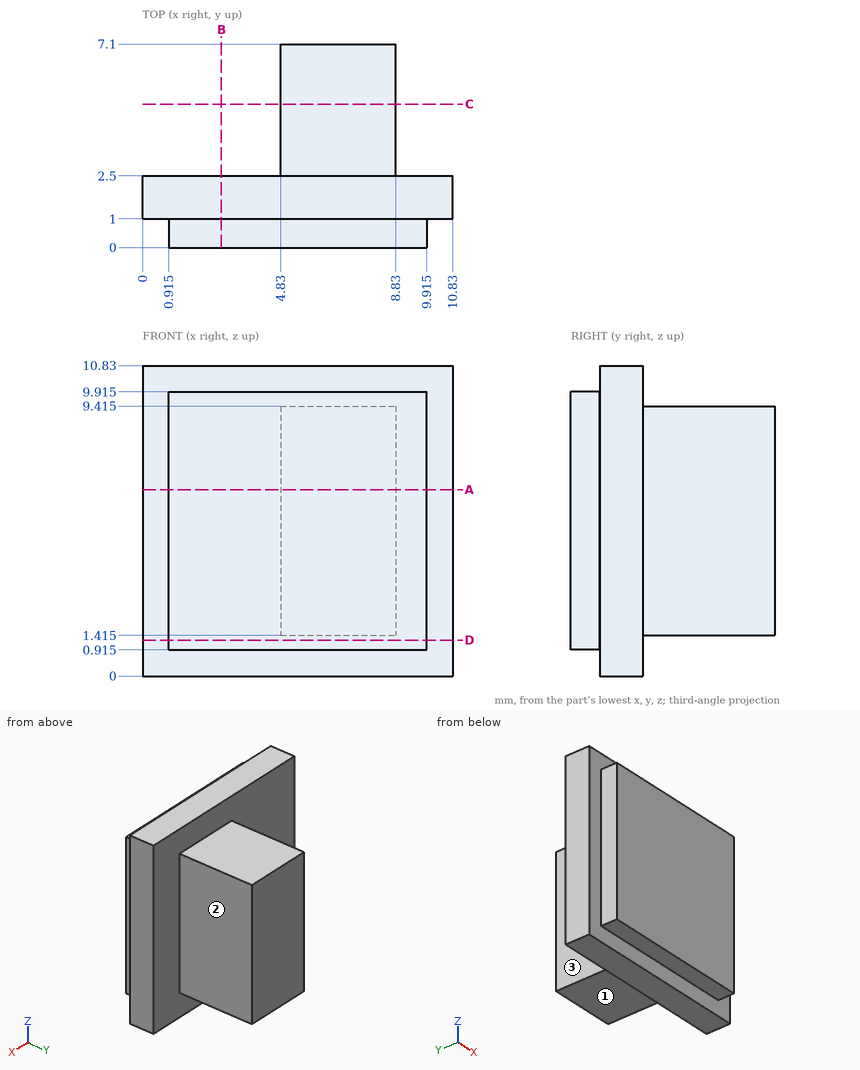
Could you check a few things on this drawing? It's one solid part, dimensions in mm from its lowest x, y, z. A direction names the side the tool comes from. Give positions to 0.01 mm unless a question says otherwise; leave off trailing zeros. Loops run counter-clockwise (first coordinate to the right, second up) from the corner with the lowest first, then second, coordinate; pieces in that order, holes last. Notation, with made-up numbers: (78.5, 44.5) -> (92.5, 44.5) arc R28 cw to (92.5, 77.5) -> close; hole circle Ø3 at (-39.75, -2.5). An arc over 180 degrees is marked (long way). Answer as CSV lines item,"result". Start each with the question number.
(1) If we section it at D-D on z = 1.25: Write out the boundary of the cut face in (x, y) (3 decimals), then the cut area to 3 significant figures.
(2) If we section it at C-C on y = 5: Write out the boundary of the cut face in (x, z) (3 decimals).
(3) Which directions (+Z, -Z, +X, -X, +Y, -Y) give clear straight access to the entire face, cutting with the end or side of a thin tool? Please do the marked faces 1, 2 and 3.
(4) If we section it at A-A on z = 6.5: Write out the boundary of the cut face in (x, y) (3 decimals), then the cut area to 3 significant figures.
(5) I'm going to push flat-ended pins straight in: pin 1 Ø1.5 at (y, z) = (3.5, 6) entering from +X; pin 2 Ø0.5 at (y, z) = (0.5, 5) entering from +X (3 decimals); pin 3 Ø0.8 at (x, y) = (5, 0.5) entering from +Z (3 decimals). Where does each tip first touch, or does it pass through?
(6) I need wall thicknesses on probe 1 along Y at (x, z) = (3, 8.75); probe 2 along Y at (x, z) = (7, 10.25); probe 3 along X at (y, z) = (5.5, 5.25). Which ranges of each line are inside material? Lowest first, please.
(7) If we section it at B-B on x = 2.75: Write out the boundary of the cut face in (y, z) (3 decimals).
Computed:
1,outline,"(0, 1) -> (0.915, 1) -> (0.915, 0) -> (9.915, 0) -> (9.915, 1) -> (10.83, 1) -> (10.83, 2.5) -> (0, 2.5) -> close"
1,area,"25.2 mm2"
2,outline,"(4.83, 1.415) -> (8.83, 1.415) -> (8.83, 9.415) -> (4.83, 9.415) -> close"
3,face 1,"-Z, +X, -X, +Y"
3,face 2,"+Z, -Z, +X, +Y"
3,face 3,"+Z, -Z, -X, +Y"
4,outline,"(0, 1) -> (0.915, 1) -> (0.915, 0) -> (9.915, 0) -> (9.915, 1) -> (10.83, 1) -> (10.83, 2.5) -> (8.83, 2.5) -> (8.83, 7.1) -> (4.83, 7.1) -> (4.83, 2.5) -> (0, 2.5) -> close"
4,area,"43.6 mm2"
5,pin 1,"stops at x = 8.83"
5,pin 2,"stops at x = 9.915"
5,pin 3,"stops at z = 9.915"
6,probe 1,"y = 0 to 2.5"
6,probe 2,"y = 1 to 2.5"
6,probe 3,"x = 4.83 to 8.83"
7,outline,"(0, 0.915) -> (1, 0.915) -> (1, 0) -> (2.5, 0) -> (2.5, 10.83) -> (1, 10.83) -> (1, 9.915) -> (0, 9.915) -> close"
